from build123d import *

# Parameters (mm, degrees)
CROQUIS1_W              = 82
CROQUIS1_H              = 144
SALIENTE_EXTRUIR1_DEPTH = 2
CROQUIS2_W              = 3
CROQUIS2_H              = 22.5
SALIENTE_EXTRUIR4_DEPTH = 24


with BuildPart() as part:
    # Croquis1 → Saliente-Extruir1 (new body)
    with BuildSketch(Plane(origin=(0, 0, 0), x_dir=(1, 0, 0), z_dir=(0, 1, 0))):
        Rectangle(CROQUIS1_W, CROQUIS1_H)
    extrude(amount=SALIENTE_EXTRUIR1_DEPTH)

    # Croquis2 → Saliente-Extruir4 (add)
    with BuildSketch(Plane.XZ):
        with Locations((39.5, 67.25)):
            Rectangle(CROQUIS2_W, CROQUIS2_H)
        with Locations((39.5, -47.75)):
            Rectangle(CROQUIS2_W, CROQUIS2_H)
    extrude(amount=-SALIENTE_EXTRUIR4_DEPTH)


solid = part.part
Read the model definition and answer for the solid it produces. Units are mm, in the model's axes. A direction names the side the tool comes from. Give positions to 0.01 mm unless a question says otherwise; leave off trailing zeros. Write each loop counter-clockwise with the first axis right and the second up, starting at its lowest first coordinate (ties: lowest second). Pieces come first, ordered by that corner, then holes. Notation, with made-up numbers: (-31, 89) - (-26, 89) arc R22 ccw to (-26, 102) - close; hole circle Ø8 at (65.25, 71.5). An arc over 180 degrees is marked (long way). Use CSV: the item, a comma, the result in double quotes. Start each with the question number.
Item 1: The part is cut by section B-B, the plane x = 12.5. Give the vertices of the cut face in (y, z), and give its area (3 significant figures).
Item 2: For faces 1 (the flat face through (39, 13, 56)), 2 (the flat face through (39, 13, -59)), 3 (the flat face through (38, 13, -48)), determine the directions among +Z, -Z, +X, -X, +Y, -Y from which every point of the face is accessible in a straight line to the end or side of a thin tool.
Item 3: The part is cut by section C-C, the plane z = -50.5. Give the vertices of the cut face in (x, y).
Item 4: Consider line 1 (Y direction, x = -7, z = -2.5); line 2 (X direction, y = 9.25, z = -44.5). Determine where each line is inside the solid, lowest interval first.
Item 5: The part is cut by section D-D, the plane z = 13.5. Give the vertices of the cut face in (x, y), and give its area (3 significant figures).
Item 6: The part is cut by section A-A, the plane y = 19.5. Give the vertices of the cut face in (x, z), and give its area (3 significant figures).
Item 7: Flat-ended cylindrical pins translate along their axes: P1, Ø1, axis at x = -5.5, z = 48, coming from the +Y side; P2, Ø2.5, axis at x = 40, y = 16, coming from the -Z side; P3, Ø6, axis at y = 19, z = 62.5, coming from the -X side. Find the tip coordinate at first contact, or state that the pin passes through.
Taken from the geometry:
1,outline,"(0, -72) - (2, -72) - (2, 72) - (0, 72) - close"
1,area,"288 mm2"
2,face 1,"+X, -X, +Y"
2,face 2,"-Z, +X, -X, +Y"
2,face 3,"+Z, -Z, -X, +Y"
3,outline,"(-41, 0) - (41, 0) - (41, 24) - (38, 24) - (38, 2) - (-41, 2) - close"
4,line 1,"0 to 2"
4,line 2,"38 to 41"
5,outline,"(-41, 0) - (41, 0) - (41, 2) - (-41, 2) - close"
5,area,"164 mm2"
6,outline,"(38, -59) - (41, -59) - (41, -36.5) - (38, -36.5) - close; (38, 56) - (41, 56) - (41, 78.5) - (38, 78.5) - close"
6,area,"135 mm2"
7,P1,"y = 2"
7,P2,"z = -59"
7,P3,"x = 38"
